Geometry check sheet. Reference: the model listing, model coordinates, mm. Coordinates: 2 decimals unless noted, no trailing zeros. Write each loop counter-clockwise with the first axis right and the second up, starting at its lowest first coordinate (ties: lowest second). Pieces come first, ordered by that corner, then holes. Notation, with made-up numbers: (37, 78) -> (65, 78) arc R20 cw to (65, 91) -> close; hole circle Ø10 at (22, 71.5). An arc over 180 degrees is marked (long way). Use a Markdown table: item, result.
```python
from build123d import *

# Parameters (mm, degrees)
F1_DEPTH = 0.8
F2_SIZE  = 2.5
F4_D     = 1.1


with BuildPart() as f1:
    # F0 (on Right) → F1 (new body, symmetric)
    with BuildSketch(Plane.YZ):
        with BuildLine():
            Line((3.4, 1), (3.4, 0))
            Line((3.4, 0), (7.4, 0))
            Line((7.4, 0), (7.4, -4.8))
            Line((7.4, -4.8), (17.4, -4.8))
            Line((17.4, -4.8), (17.4, -2.1))
            Line((17.4, -2.1), (23.3, -2.1))
            Line((23.3, -2.1), (23.3, -4.8))
            Line((23.3, -4.8), (33.3, -4.8))
            Line((33.3, -4.8), (33.3, 0))
            Line((33.3, 0), (50.4, 0))
            Line((50.4, 0), (49.1, 2.2))
            Line((49.1, 2.2), (1.2466947794, 16.278038907))
            ThreePointArc((1.2466947794, 16.278038907), (-1.3972083437, 15.8020912075), (-2.6, 13.4))
            Line((-2.6, 13.4), (-2.6, 7))
            ThreePointArc((-2.6, 7), (-1.7213203436, 4.8786796564), (0.4, 4))
            ThreePointArc((0.4, 4), (2.5213203436, 3.1213203436), (3.4, 1))
        make_face()
    extrude(amount=F1_DEPTH, both=True)

    # F2
    f2_edges = [f1.edges().sort_by_distance(p)[0] for p in [
        (0, 7.4, -4.8),
        (0, 23.3, -4.8),
        (0, 17.4, -4.8),
        (0, 33.3, -4.8),
    ]]
    chamfer(f2_edges, length=F2_SIZE)

    # F4 (through all)
    with Locations(Plane.YZ.offset(0.8)):
        with Locations((0, 14), (0, 11), (0, 8)):
            Hole(F4_D / 2)


solid = f1.part
```
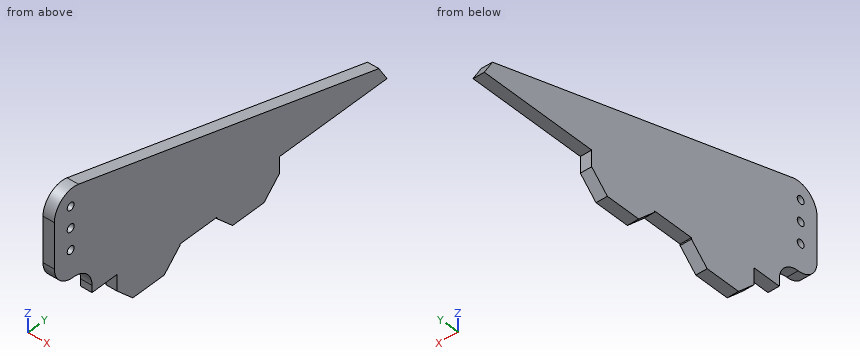
Item 1: Section check C-C on z = 14. Record the boundary of the cut face in (x, y).
Answer block:
| item | result |
|---|---|
| outline | (-0.8, -2.54) -> (0.8, -2.54) -> (0.8, -0.55) -> (-0.8, -0.55) -> close; (-0.8, 0.55) -> (0.8, 0.55) -> (0.8, 8.99) -> (-0.8, 8.99) -> close |
Item 2: Section check A-A on x = -0.3. Record the boundary of the cut face in (y, z).
Answer block:
| item | result |
|---|---|
| outline | (-2.6, 7) arc R3 ccw to (0.4, 4) arc R3 cw to (3.4, 1) -> (3.4, 0) -> (7.4, 0) -> (7.4, -2.3) -> (9.9, -4.8) -> (14.9, -4.8) -> (17.4, -2.3) -> (17.4, -2.1) -> (23.3, -2.1) -> (23.3, -2.3) -> (25.8, -4.8) -> (30.8, -4.8) -> (33.3, -2.3) -> (33.3, 0) -> (50.4, 0) -> (49.1, 2.2) -> (1.25, 16.28) arc R3 ccw to (-2.6, 13.4) -> close; hole circle Ø1.1 at (0, 8); hole circle Ø1.1 at (0, 11); hole circle Ø1.1 at (0, 14) |
Item 3: Thickness scan on L1, parallel to Z at x = -0.15, y = 0; L2, parallel to Y at x = 0.7, z = -2.25; L3, parallel to Z at x = -0.1, y = 12. Record the ranges inside material, lowest first. Write a range as [from, to].
Answer block:
| item | result |
|---|---|
| L1 | z = [4.03, 7.45], [8.55, 10.45], [11.55, 13.45], [14.55, 16.37] |
| L2 | y = [7.4, 17.4], [23.3, 33.3] |
| L3 | z = [-4.8, 13.11] |
Item 4: Section check D-D on y = 37. Record the boundary of the cut face in (x, z).
Answer block:
| item | result |
|---|---|
| outline | (-0.8, 0) -> (0.8, 0) -> (0.8, 5.76) -> (-0.8, 5.76) -> close |
Item 5: Section check B-B on z = 11. Record the boundary of the cut face in (x, y), then the cut area to 3 significant figures.
Answer block:
| item | result |
|---|---|
| outline | (-0.8, -2.6) -> (0.8, -2.6) -> (0.8, -0.55) -> (-0.8, -0.55) -> close; (-0.8, 0.55) -> (0.8, 0.55) -> (0.8, 19.19) -> (-0.8, 19.19) -> close |
| area | 33.1 mm^2 |
Item 6: Depth check by flat-ended pin: P1, Ø0.8, axis at x = 0, z = -0.5, coming from the +Y side; P2, Ø0.8, axis at x = 0.5, z = 0.5, coming from the -Y side; P3, Ø0.8, axis at x = -0.5, y = 5, coming from the -Z side. Enter the tip coordinate at first touch or a pass-through.
Answer block:
| item | result |
|---|---|
| P1 | stops at y = 33.3 |
| P2 | stops at y = 3.4 |
| P3 | stops at z = 0 |
